```python
from build123d import *

# Parameters (mm, degrees)
F0_R     = 15
F2_W     = 25
F2_H     = 25
F4_R     = 3
F5_R     = 5
F6_DEPTH = 1.5
F7_R     = 4
F8_DEPTH = 20


with BuildPart() as f3:
    # F0 (on Top) → F3 section 0
    with BuildSketch(Plane.XY):
        Circle(F0_R)
    # F2 (on offset) → F3 section 1
    with BuildSketch(Plane.XY.offset(89.4)):
        Rectangle(F2_W, F2_H)
    loft()

    # F4
    f4_edges = [f3.edges().sort_by_distance(p)[0] for p in [
        (12.5, 6.25, 89.4),
        (12.5, -6.25, 89.4),
        (0, 12.5, 89.4),
        (-12.5, 0, 89.4),
        (0, -12.5, 89.4),
    ]]
    fillet(f4_edges, radius=F4_R)

    # F5 (on Right) → F6 (join, symmetric)
    with BuildSketch(Plane.YZ):
        with BuildLine():
            Line((9.5, 83.3456217407), (9.5, 105.2605534294))
            ThreePointArc((9.5, 105.2605534294), (0, 95.7605534294), (-9.5, 105.2605534294))
            Line((-9.5, 105.2605534294), (-9.5, 83.3456217407))
            Line((-9.5, 83.3456217407), (9.5, 83.3456217407))
        make_face()
        with BuildLine():
            ThreePointArc((-9.5, 105.2605534294), (0, 95.7605534294), (9.5, 105.2605534294))
            ThreePointArc((9.5, 105.2605534294), (0, 114.7605534294), (-9.5, 105.2605534294))
        make_face()
        with Locations((0, 105.2605534294)):
            Circle(F5_R, mode=Mode.SUBTRACT)
    extrude(amount=F6_DEPTH, both=True)

    # F7 (on Top) → F8 (cut)
    with BuildSketch(Plane.XY):
        Circle(F7_R)
    extrude(amount=F8_DEPTH, mode=Mode.SUBTRACT)


solid = f3.part
```
Read the model definition and answer for the solid it produces. Units are mm, in the model's axes. A direction names the side the tool comes from. Coordinates: 2 decimals unless noted, no trailing zeros. Write each loop counter-clockwise with the first axis right and the second up, starting at its lowest first coordinate (ties: lowest second). Pieces come first, ordered by that corner, then holes. Notation, with made-up numbers: (77, -12) -> (107, -12) arc R7 ccw to (107, -7) -> close; hole circle Ø5 at (-37, -3). An arc over 180 degrees is marked (long way). Answer as a JSON object with one key per item and string values.
Q1. Determine the mould class of faces 1 (the cylindrical face through (-0.867, -3.905, 9.86)), 2 (the flat face through (1.5, 0, 99)), 3 (the flat face through (-1.5, 0, 99)), 4 (the flat face through (0, 0, 20)) for opening direction X: pulls with the +X half, pulls with the -X half, needs draft (parallel to the pull), parting line crosses it, or undercut.
The answers:
{"face 1": "undercut", "face 2": "pulls with the +X half", "face 3": "pulls with the -X half", "face 4": "undercut"}
Q2. A tool of negligible diameter and unlimited length cuts with its end or side. For faces 5 (the flat face through (0, -9.5, 97)), 6 (the cylindrical face through (0.02, 0.21, 114.76)), 7 (the flat face through (0, 9.5, 97)), from which of +Z, -Z, +X, -X, +Y, -Y can it reach the whole face along a straight path? Write none if from no direction.
The answers:
{"face 5": "+Z, +X, -X, -Y", "face 6": "+Z, +X, -X", "face 7": "+Z, +X, -X, +Y"}
Q3. Flat-ended cylindrical pins translate along their axes: pin 1 Ø12 at (x, z) = (-4, 87) entering from +Y; pin 2 Ø2 at (y, z) = (-2, 102) entering from +X; pin 3 Ø8 at (y, z) = (-8.5, 77) entering from -X; pin 4 Ø1 at (x, y) = (-5.5, 2.5) entering from +Z. Find the tip coordinate at first contact, or state that the pin passes through.
The answers:
{"pin 1": "stops at y = 12.71", "pin 2": "passes through", "pin 3": "stops at x = -12.78", "pin 4": "stops at z = 89.4"}
Q4. The part is cut by section A-A on z = 104. Give the vertices of the cut face in (x, y), then the cut area to 3 significant figures.
The answers:
{"outline": "(-1.5, -9.5) -> (1.5, -9.5) -> (1.5, -4.84) -> (-1.5, -4.84) -> close; (-1.5, 4.84) -> (1.5, 4.84) -> (1.5, 9.5) -> (-1.5, 9.5) -> close", "area": "28.0 mm2"}
Q5. Consider line 1 (Z direction, x = 0, y = 0); line 2 (X direction, y = -7, z = 90); line 3 (Z direction, x = -3, y = -2). Determine where each line is inside the solid, lowest interval first. Write a range as [from, to].
The answers:
{"line 1": "z = [20, 100.26], [110.26, 114.76]", "line 2": "x = [-1.5, 1.5]", "line 3": "z = [20, 89.4]"}
